```python
from build123d import *

# Parameters (mm, degrees)
SKETCH1_W                                       = 77.3
SKETCH1_H                                       = 32.2
BOSS_EXTRUDE1_DEPTH                             = 2.5
SKETCH3_W                                       = 77.3
SKETCH3_H                                       = 5.2
BOSS_EXTRUDE2_DEPTH                             = 28.599
FILLET1_R                                       = 2.5
SKETCH4_W                                       = 77.3
SKETCH4_H                                       = 37.342788029
CUT_REVOLVE2_ANGLE                              = 3
CSK_FOR_M5_FLAT_HEAD_MACHINE_SCREW1_D           = 5.5
CSK_FOR_M5_FLAT_HEAD_MACHINE_SCREW1_DEPTH       = 12.4
CSK_FOR_M5_FLAT_HEAD_MACHINE_SCREW1_CSINK_D     = 10.4
CSK_FOR_M5_FLAT_HEAD_MACHINE_SCREW1_CSINK_ANGLE = 90
CSK_FOR_M5_FLAT_HEAD_MACHINE_SCREW1_TIP         = 1.652366702


with BuildPart() as part:
    # Sketch1 → Boss-Extrude1 (new body)
    with BuildSketch(Plane.XY):
        Rectangle(SKETCH1_W, SKETCH1_H)
    extrude(amount=BOSS_EXTRUDE1_DEPTH)

    # Sketch3 → Boss-Extrude2 (add)
    with BuildSketch(Plane.XY.offset(2.5)):
        with Locations((0, 13.5)):
            Rectangle(SKETCH3_W, SKETCH3_H)
    extrude(amount=BOSS_EXTRUDE2_DEPTH)

    # Fillet1
    fillet1_edges = [part.edges().sort_by_distance(p)[0] for p in [
        (-38.65, 13.5, 31.099),
        (38.65, 13.5, 31.099),
    ]]
    fillet(fillet1_edges, radius=FILLET1_R)

    # Sketch4 → Cut-Revolve2 (revolve, cut)
    with BuildSketch(Plane(origin=(0, 16.1, 0), x_dir=(1, 0, 0), z_dir=(0, 1, 0))):
        with Locations((0, -18.671394015)):
            Rectangle(SKETCH4_W, SKETCH4_H)
    revolve(axis=Axis((-38.65, 16.1, 0), (1, 0, 0)), revolution_arc=CUT_REVOLVE2_ANGLE, mode=Mode.SUBTRACT)

    # CSK for M5 Flat Head Machine Screw1
    with Locations(Plane(origin=(0, 0, 0), x_dir=(-1, 0, 0), z_dir=(0, 0, -1))):
        with Locations((-28.65, -4), (28.65, -4)):
            CounterSinkHole(CSK_FOR_M5_FLAT_HEAD_MACHINE_SCREW1_D / 2, CSK_FOR_M5_FLAT_HEAD_MACHINE_SCREW1_CSINK_D / 2, depth=CSK_FOR_M5_FLAT_HEAD_MACHINE_SCREW1_DEPTH, counter_sink_angle=CSK_FOR_M5_FLAT_HEAD_MACHINE_SCREW1_CSINK_ANGLE)
            with Locations((0, 0, -(CSK_FOR_M5_FLAT_HEAD_MACHINE_SCREW1_DEPTH + CSK_FOR_M5_FLAT_HEAD_MACHINE_SCREW1_TIP / 2))):  # 118° drill point
                Cone(0, CSK_FOR_M5_FLAT_HEAD_MACHINE_SCREW1_D / 2, CSK_FOR_M5_FLAT_HEAD_MACHINE_SCREW1_TIP, mode=Mode.SUBTRACT)


solid = part.part
```
Here's how the part is built. I have some questions about the finished solid (model axes, mm). A direction names the side the tool comes from. Round coordinates to 2 decimals unless told otherwise and drop trailing zeros. Order: outer loops, then holes, each group sorted by start corner. A loop starts at its lowest first (then second) coordinate and runs counter-clockwise, first axis right, second up. Notation, with made-up numbers: M 49,-1.5 L 73,-1.5 A20 ccw 73,26.5 Z; hole C 24,-37.75 d11. An arc over 180 degrees is marked long. Use CSV: the item, a comma, the result in double quotes.
1) If we mould it in two halves opening along X, with no side actions, what happens to faces 1 (the conical face through (-30.765, -2.061, 2.331)), 2 (the flat face through (-38.65, 12, 10)), 3 (the flat face through (-1, -2, 2.5)), 4 (the conical face through (31.3, -5.1, 2.33))? For each: pulls with the +X half, pulls with the -X half, needs draft (parallel to the pull), parting line crosses it, or undercut.
Taken from the geometry:
face 1,"undercut"
face 2,"pulls with the -X half"
face 3,"needs draft"
face 4,"undercut"
2) I need wall thicknesses on line 1 along X through (y, z) = (-4, 2); line 2 along Z through (x, y) = (-34, -1); line 3 along Y through (x, z) = (28, 2). Which ranges of each line are inside material? Lowest first, please. Write a range as [from, to].
Taken from the geometry:
line 1,"[-38.65, -31.85], [-25.45, 25.45], [31.85, 38.65]"
line 2,"[0, 2.5]"
line 3,"[-16.1, -7.13], [-0.87, 16]"
3) I'm going to push flat-ended pins straight in: P1, Ø4, axis at x = -20, z = 12.5, coming from the +Y side; P2, Ø2, axis at x = -24.5, y = 3, coming from the +Z side; P3, Ø9, axis at x = -28.65, y = -4, coming from the -Z side. Where does each tip first touch, or does it pass through?
Taken from the geometry:
P1,"y = 15.55"
P2,"z = 2.5"
P3,"z = 0.7"
4) I want a section at D-D (z = 25.5). List the corners of the cut face in (x, y) for me.
Taken from the geometry:
outline,"M -38.65,10.9 L 38.65,10.9 L 38.65,14.76 L -38.65,14.76 Z"
5) On a 3-axis mill with a long thin cutter (end or side, diameter ignored), from which of +Z, -Z, +X, -X, +Y, -Y can I reach the whole of each face in a straight line? I mean faces 5 (the flat face through (-1, 10.9, 17)), 6 (the cylindrical face through (37.937, 12.777, 30.347)). Say none if no direction works.
Taken from the geometry:
face 5,"+Z, +X, -X, -Y"
face 6,"+Z, +X, +Y, -Y"
6) I want a section at C-C (x = 3). List the corners of the cut face in (y, z) for me.
Taken from the geometry:
outline,"M -16.1,0 L 16.1,0 L 14.47,31.1 L 10.9,31.1 L 10.9,2.5 L -16.1,2.5 Z"
7) I want a section at A-A (y = -4). List the corners of the cut face in (x, z) for me, then the cut area to 3 significant figures.
Taken from the geometry:
outline,"M -38.65,0 L -33.85,0 L -31.4,2.45 L -31.4,2.5 L -38.65,2.5 Z; M -25.9,2.45 L -23.45,0 L 23.45,0 L 25.9,2.45 L 25.9,2.5 L -25.9,2.5 Z; M 31.4,2.45 L 33.85,0 L 38.65,0 L 38.65,2.5 L 31.4,2.5 Z"
area,"154 mm^2"
8) I want a section at B-B (x = 28.65). List the corners of the cut face in (y, z) for me.
Taken from the geometry:
outline,"M -16.1,0 L -9.2,0 L -6.75,2.45 L -6.75,2.5 L -16.1,2.5 Z; M -1.25,2.45 L 1.2,0 L 16.1,0 L 14.47,31.1 L 10.9,31.1 L 10.9,2.5 L -1.25,2.5 Z"
